from build123d import *

# Parameters (mm, degrees)
SKETCH_R     = 5
PAD_DEPTH    = 14
PAD001_DEPTH = 27


with BuildPart() as part:
    # Sketch → Pad (new body)
    with BuildSketch(Plane.XY):
        with BuildLine():
            Line((0, 34.821453), (75.88228, 14.488889))
            ThreePointArc((75.88228, -14.488889), (87, 0), (75.88228, 14.488889))
            Line((0, -34.821453), (75.88228, -14.488889))
            Line((0, -15), (0, -34.821453))
            ThreePointArc((0, -15), (15, 0), (0, 15))
            Line((0, 34.821453), (0, 15))
        make_face()
        with Locations((72, 0)):
            Circle(SKETCH_R, mode=Mode.SUBTRACT)
    extrude(amount=PAD_DEPTH)

    # Sketch001 (on Face9 of Pad) → Pad001 (join)
    with BuildSketch(Plane.XY.offset(14)):
        with BuildLine():
            ThreePointArc((0, -33.634944), (33.634944, 0), (0, 33.634944))
            Line((0, 15), (0, 33.634944))
            ThreePointArc((0, -15), (15, 0), (0, 15))
            Line((0, -15), (0, -33.634944))
        make_face()
    extrude(amount=PAD001_DEPTH)

    # Mirrored: part across YZ


with BuildPart() as part_1:
    add(part.part)
    add(part.part.mirror(Plane.YZ))


solid = part_1.part
Build history of the part. All positions in model axes, mm. A direction names the side the tool comes from. Round coordinates to 2 decimals unless told otherwise and drop trailing zeros. Write each loop counter-clockwise with the first axis right and the second up, starting at its lowest first coordinate (ties: lowest second). Pieces come first, ordered by that corner, then holes. Notation, with made-up numbers: (57.5, 41.5) - (86.5, 41.5) arc R17 ccw to (86.5, 72.5) - close; hole circle Ø7 at (77.5, 8.25). An arc over 180 degrees is marked (long way). One line per question, with ' | ' between items.
1. Drop flat-ended pins along their axis: pin 1 Ø3 at (x, z) = (66.5, 6) entering from -Y; pin 2 Ø19.5 at (x, y) = (56, -16) entering from +Z; pin 3 Ø1 at (y, z) = (13.5, 4.5) entering from +X; pin 4 Ø24 at (x, y) = (0, 0) entering from +Z. Give the stop position or say it passes through.
Results are:
pin 1: y = -17.4 | pin 2: z = 14 | pin 3: x = 79.48 | pin 4: through
2. Drill centre lines: line 1 along X through (y, z) = (-1.5, 11.5); line 2 along X through (y, z) = (0, 21); line 3 along Z through (x, y) = (-71, -9). Where is each one in solid material? Low to high. Write a range as from..to.
Results are:
line 1: -86.92..-76.77, -67.23..-14.92, 14.92..67.23, 76.77..86.92 | line 2: -33.63..-15, 15..33.63 | line 3: 0..14
3. Band-saw the part on B-B, the plane z = 6. Write the cut outline in (x, y).
Results are:
outline: (-75.88, -14.49) - (0, -34.82) - (75.88, -14.49) arc R15 ccw to (75.88, 14.49) - (0, 34.82) - (-75.88, 14.49) arc R15 ccw to start; hole circle Ø10 at (-72, 0); hole circle Ø30 at (0, 0); hole circle Ø10 at (72, 0)
4. Band-saw the part on C-C, the plane x = 2.5. Write the cut outline in (y, z), and give its area (3 significant figures).
Results are:
outline: (-34.15, 0) - (-14.79, 0) - (-14.79, 41) - (-33.54, 41) - (-33.54, 14) - (-34.15, 14) - close; (14.79, 0) - (34.15, 0) - (34.15, 14) - (33.54, 14) - (33.54, 41) - (14.79, 41) - close | area: 1,550 mm^2
5. Tool access for faces 1 (the face through (-10.103, -32.082, 27.311)), 2 (the face through (-14, -7, 41)): list every direction of +Z, -Z, +X, -X, +Y, -Y with a clear straight run to the whole face (end or side of a thin tool).
Results are:
face 1: +Z | face 2: +Z, +X, -X, +Y, -Y
6. Band-saw the part on A-A, the plane y = 0. Write the cut outline in (x, z), and give its area (3 significant figures).
Results are:
outline: (-87, 0) - (-77, 0) - (-77, 14) - (-87, 14) - close; (-67, 0) - (-15, 0) - (-15, 41) - (-33.63, 41) - (-33.63, 14) - (-67, 14) - close; (15, 0) - (67, 0) - (67, 14) - (33.63, 14) - (33.63, 41) - (15, 41) - close; (77, 0) - (87, 0) - (87, 14) - (77, 14) - close | area: 2,740 mm^2
7. Band-saw the part on D-D, the plane z = 35. Write the cut outline in (x, y).
Results are:
outline: circle Ø67.27 at (0, 0); hole circle Ø30 at (0, 0)
